Verification items for this drawing (mm, ordinates from the low corner). A direction names the side the tool comes from. Round coordinates to 2 decimals unless told otherwise and drop trailing zeros. Loops run counter-clockwise (first coordinate to the right, second up) from the corner with the lowest first, then second, coordinate; pieces in that order, holes last. Notation, with made-up numbers: (64.25, -20.5) - (118.25, -20.5) arc R21 cw to (118.25, -3.5) - close; hole circle Ø9 at (53, 80.5). An arc over 180 degrees is marked (long way). Write item = value, one per line.
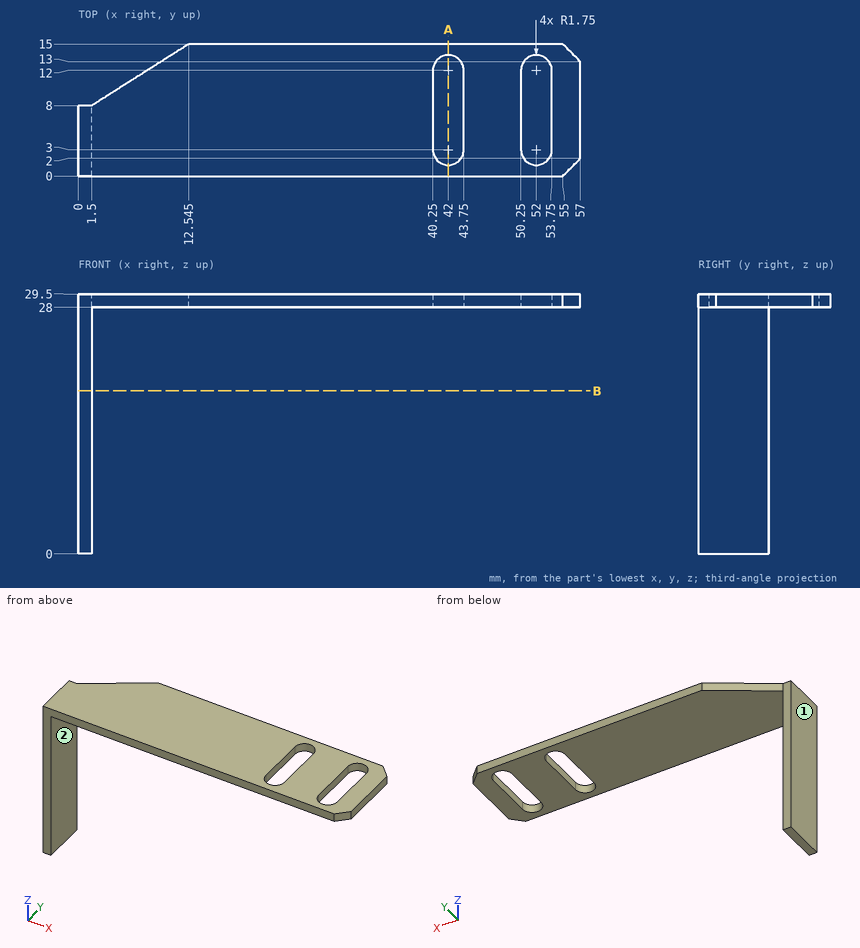
(1) Scan lines: L1, parallel to Z at x = 34.5, y = 6.25; L2, parallel to X at y = 7.5, z = 26.75. Record each from-to range of solid material in increasing order. Write a range as [from, to].
Answers follow:
L1 = [28, 29.5]
L2 = [0, 1.5]
(2) Set-up check for the marked faces 1 and 2: record each of +Z, -Z, +X, -X, +Y, -Y from which the full face is reachable in a straight line by a thin tool's end or side.
Answers follow:
face_1 = +Z, -Z, -X, +Y, -Y
face_2 = -Z, +X, +Y, -Y
(3) Section check B-B (z = 18.5). Enter the section's corners in (x, y).
Answers follow:
outline = (0, 0) - (1.5, 0) - (1.5, 8) - (0, 8) - close
(4) Gauge pin test, flat ends, axial feed: pin 1 (8 mm diameter, centred on x = 27.5, y = 12.5, fed in from -Z); pin 2 (2.5 mm diameter, centred on y = 5, z = 20, fed in from +X). Record the tip position at first contact, or that the pin passes through.
Answers follow:
pin_1 = 28
pin_2 = 1.5
(5) Section check A-A (x = 42). Enter the section's corners in (y, z).
Answers follow:
outline = (0, 28) - (1.25, 28) - (1.25, 29.5) - (0, 29.5) - close; (13.75, 28) - (15, 28) - (15, 29.5) - (13.75, 29.5) - close
